The listing builds one solid part. Answer for the finished solid, in the listing's coordinates (mm). A direction names the side the tool comes from. Coordinates: 2 decimals unless noted, no trailing zeros. Order: outer loops, then holes, each group sorted by start corner. A loop starts at its lowest first (then second) coordinate and runs counter-clockwise, first axis right, second up. Notation, with made-up numbers: (51, 14.5) -> (60, 14.5) arc R17 ccw to (60, 42.5) -> close; hole circle Ø1 at (17.25, -37). An arc over 180 degrees is marked (long way). Put each result on its own line as item: value. Start each with the question number.
```python
from build123d import *

# Parameters (mm, degrees)
SALIENTE_EXTRUIR1_DEPTH                              = 100
CROQUIS3_W                                           = 20.92
CROQUIS3_H                                           = 92
CORTAR_EXTRUIR1_DEPTH                                = 798
CROQUIS4_W                                           = 19.08
CROQUIS4_H                                           = 92
CROQUIS4_W_2                                         = 20.25
CORTAR_EXTRUIR2_DEPTH                                = 798
CROQUIS5_W                                           = 465.67
CROQUIS5_H                                           = 136.54
CORTAR_EXTRUIR3_DEPTH                                = 69
REFRENTADO_PARA_PERNO_CON_CABEZA_HEXAGON_D           = 10.5
REFRENTADO_PARA_PERNO_CON_CABEZA_HEXAGON_DEPTH       = 90
REFRENTADO_PARA_PERNO_CON_CABEZA_HEXAGON_CBORE_D     = 13
REFRENTADO_PARA_PERNO_CON_CABEZA_HEXAGON_CBORE_DEPTH = 6.85
REFRENTADO_PARA_PERNO_CON_CABEZA_HEXAGON_TIP         = 3.15451825
CROQUIS8_R                                           = 8.5
CORTAR_EXTRUIR4_DEPTH                                = 69
CORTAR_EXTRUIR5_DEPTH                                = 607
CORTAR_EXTRUIR6_START                                = -138.5400001
CORTAR_EXTRUIR6_DEPTH                                = 138.5400001
REDONDEO1_R                                          = 10
REDONDEO2_R                                          = 10
REDONDEO3_R                                          = 10
REDONDEO4_R                                          = 10
REDONDEO5_R                                          = 10
CHAFL_N1_SIZE                                        = 1
REDONDEO6_R                                          = 10
SALIENTE_EXTRUIR2_DEPTH                              = 61
CROQUIS12_R                                          = 6.5
CORTAR_EXTRUIR7_DEPTH                                = 61
CORTAR_EXTRUIR8_DEPTH                                = 630
CORTAR_EXTRUIR9_START                                = -630
CROQUIS14_R                                          = 8.5
CORTAR_EXTRUIR9_DEPTH                                = 630


# Read off the part's stored shape, not the designer's step: Cortar-Extruir6
# Some blends are built 0.0001 mm under size
with BuildPart() as part:
    # Croquis2 → Saliente-Extruir1 (new body)
    with BuildSketch(Plane(origin=(0, 0, 0), x_dir=(1, 0, 0), z_dir=(0, 1, 0))):
        Polygon((-10, 20.92), (-10, 181.28), (497, 181.28), (497, 14.25), (482, 14.25), (482, 0), (0, 0), (0, 20.92), align=None)
    extrude(amount=SALIENTE_EXTRUIR1_DEPTH)

    # Croquis3 → Cortar-Extruir1 (cut)
    with BuildSketch(Plane.ZY.offset(10)):
        Polygon((-181.28, 100), (-181.28, 8), (-159.46, 8), (-159.46, 100), (-159.605192294, 100), align=None)
        with Locations((-10.46, 54)):
            Rectangle(CROQUIS3_W, CROQUIS3_H)
    extrude(amount=-CORTAR_EXTRUIR1_DEPTH, mode=Mode.SUBTRACT)

    # Croquis4 → Cortar-Extruir2 (cut)
    with BuildSketch(Plane(origin=(0, 0, -159.46), x_dir=(-1, 0, 0), z_dir=(0, 0, -1))):
        with Locations((0.46, 54)):
            Rectangle(CROQUIS4_W, CROQUIS4_H)
        with Locations((-486.875, 54)):
            Rectangle(CROQUIS4_W_2, CROQUIS4_H)
    extrude(amount=-CORTAR_EXTRUIR2_DEPTH, mode=Mode.SUBTRACT)

    # Croquis5 → Cortar-Extruir3 (cut)
    with BuildSketch(Plane.XZ):
        with Locations((242.915, -90.19)):
            Rectangle(CROQUIS5_W, CROQUIS5_H)
    extrude(amount=-CORTAR_EXTRUIR3_DEPTH, mode=Mode.SUBTRACT)

    # Refrentado para perno con cabeza hexagonal de M101
    with Locations(Plane(origin=(-0.5, 8, -131.28), x_dir=(0, 0, 1), z_dir=(0, 1, 0))):
        with Locations((0, 0), (75.36, 0), (121.325, 30.5), (121.325, 140.5), (121.325, 257.25), (121.325, 368.25), (121.325, 467.5), (-40.125, 467.5), (-40.125, 368.25), (-40.125, 257.25), (-40.125, 140.5), (-40.125, 30.5)):
            CounterBoreHole(REFRENTADO_PARA_PERNO_CON_CABEZA_HEXAGON_D / 2, REFRENTADO_PARA_PERNO_CON_CABEZA_HEXAGON_CBORE_D / 2, REFRENTADO_PARA_PERNO_CON_CABEZA_HEXAGON_CBORE_DEPTH, depth=REFRENTADO_PARA_PERNO_CON_CABEZA_HEXAGON_DEPTH)
            with Locations((0, 0, -(REFRENTADO_PARA_PERNO_CON_CABEZA_HEXAGON_DEPTH + REFRENTADO_PARA_PERNO_CON_CABEZA_HEXAGON_TIP / 2))):  # 118° drill point
                Cone(0, REFRENTADO_PARA_PERNO_CON_CABEZA_HEXAGON_D / 2, REFRENTADO_PARA_PERNO_CON_CABEZA_HEXAGON_TIP, mode=Mode.SUBTRACT)

    # Croquis8 → Cortar-Extruir4 (cut)
    with BuildSketch(Plane(origin=(476.75, 0, 0), x_dir=(0, 0, -1), z_dir=(1, 0, 0))):
        with Locations((50.94, 22)):
            Circle(CROQUIS8_R)
        with Locations((136.94, 22)):
            Circle(CROQUIS8_R)
    extrude(amount=-CORTAR_EXTRUIR4_DEPTH, mode=Mode.SUBTRACT)

    # Croquis9 → Cortar-Extruir5 (cut)
    with BuildSketch(Plane(origin=(476.75, 0, 0), x_dir=(0, 0, -1), z_dir=(1, 0, 0))):
        with BuildLine():
            Line((20.92, 69), (20.92, 100))
            Line((20.92, 100), (69.776934001, 100))
            ThreePointArc((69.776934001, 100), (40.845981718, 91.596052461), (20.92, 69))
        make_face()
        with BuildLine():
            Line((110.603065999, 100), (159.46, 100))
            Line((159.46, 100), (159.46, 69))
            ThreePointArc((159.46, 69), (139.534018282, 91.596052461), (110.603065999, 100))
        make_face()
    extrude(amount=-CORTAR_EXTRUIR5_DEPTH, mode=Mode.SUBTRACT)

    # Cortar-Extruir6 outline → Cortar-Extruir6 (cut)
    with BuildSketch(Plane.XY.offset(-20.92).offset(CORTAR_EXTRUIR6_START)):
        with BuildLine():
            Line((476.75, 100), (444.284633839, 100))
            ThreePointArc((444.284633839, 100), (466.729009526, 91.005318547), (476.75, 69))
            Line((476.75, 69), (476.75, 100))
        make_face()
        with BuildLine():
            ThreePointArc((9.08, 69), (19.100990474, 91.005318547), (41.545366161, 100))
            Line((41.545366161, 100), (9.08, 100))
            Line((9.08, 100), (9.08, 69))
        make_face()
    extrude(amount=CORTAR_EXTRUIR6_DEPTH, mode=Mode.SUBTRACT)

    # Redondeo1
    redondeo1_edges = [part.edges().sort_by_distance(p)[0] for p in [
        (475.75, 69, -90.19),
        (242.915, 69, -158.46),
        (10.08, 69, -90.19),
        (242.915, 69, -21.92),
    ]]
    fillet(redondeo1_edges, radius=REDONDEO1_R)

    # Redondeo2
    # the kernel refuses this fillet: 10 mm, written as the material it adds along each edge
    with BuildSketch(Plane(origin=(20.08, 59, -31.92), x_dir=(-1, 0, 0), z_dir=(0, 0, 1))) as redondeo2_piece_1_section:
        Polygon((0, 0), (REDONDEO2_R, 0), (REDONDEO2_R, -REDONDEO2_R), (0, -REDONDEO2_R), align=None)
    redondeo2_piece_1 = extrude(amount=REDONDEO2_R, mode=Mode.PRIVATE)
    redondeo2_piece_1 = redondeo2_piece_1 - Plane(origin=(20.08, 59, -31.92), x_dir=(0.7071067811865475, -0.7071067811865475, 0), z_dir=(0, 0, 1)) * Sphere(REDONDEO2_R, mode=Mode.PRIVATE)
    add(redondeo2_piece_1)
    with BuildSketch(Plane(origin=(10.08, 0, -21.92), x_dir=(1, 0, 0), z_dir=(0, 1, 0))) as redondeo2_piece_2:
        with BuildLine():
            CenterArc((REDONDEO2_R, REDONDEO2_R), REDONDEO2_R, 180, 90)
            Line((0, REDONDEO2_R), (0, 0))
            Line((0, 0), (REDONDEO2_R, 0))
        make_face()
    extrude(amount=59)

    # Redondeo3
    # the kernel refuses this fillet: 10 mm, written as the material it adds along each edge
    with BuildSketch(Plane(origin=(465.75, 59, -31.92), x_dir=(1, 0, 0), z_dir=(0, 0, 1))) as redondeo3_piece_1_section:
        Polygon((0, 0), (REDONDEO3_R, 0), (REDONDEO3_R, REDONDEO3_R), (0, REDONDEO3_R), align=None)
    redondeo3_piece_1 = extrude(amount=REDONDEO3_R, mode=Mode.PRIVATE)
    redondeo3_piece_1 = redondeo3_piece_1 - Plane(origin=(465.75, 59, -31.92), x_dir=(-0.7071067811865475, -0.7071067811865475, 0), z_dir=(0, 0, 1)) * Sphere(REDONDEO3_R, mode=Mode.PRIVATE)
    add(redondeo3_piece_1)
    with BuildSketch(Plane(origin=(475.75, 0, -21.92), x_dir=(-1, 0, 0), z_dir=(0, 1, 0))) as redondeo3_piece_2:
        with BuildLine():
            CenterArc((REDONDEO3_R, -REDONDEO3_R), REDONDEO3_R, 90, 90)
            Line((0, -REDONDEO3_R), (0, 0))
            Line((0, 0), (REDONDEO3_R, 0))
        make_face()
    extrude(amount=59)

    # Redondeo4
    # the kernel refuses this fillet: 10 mm, written as the material it adds along each edge
    with BuildSketch(Plane(origin=(465.75, 59, -148.46), x_dir=(0, 0, -1), z_dir=(1, 0, 0))) as redondeo4_piece_1_section:
        Polygon((0, 0), (REDONDEO4_R, 0), (REDONDEO4_R, REDONDEO4_R), (0, REDONDEO4_R), align=None)
    redondeo4_piece_1 = extrude(amount=REDONDEO4_R, mode=Mode.PRIVATE)
    redondeo4_piece_1 = redondeo4_piece_1 - Plane(origin=(465.75, 59, -148.46), x_dir=(0, -0.7071067811865475, 0.7071067811865475), z_dir=(1, 0, 0)) * Sphere(REDONDEO4_R, mode=Mode.PRIVATE)
    add(redondeo4_piece_1)
    with BuildSketch(Plane(origin=(475.75, 0, -158.46), x_dir=(0, 0, 1), z_dir=(0, 1, 0))) as redondeo4_piece_2:
        with BuildLine():
            CenterArc((REDONDEO4_R, -REDONDEO4_R), REDONDEO4_R, 90, 90)
            Line((0, -REDONDEO4_R), (0, 0))
            Line((0, 0), (REDONDEO4_R, 0))
        make_face()
    extrude(amount=59)

    # Redondeo5
    # the kernel refuses this fillet: 10 mm, written as the material it adds along each edge
    with BuildSketch(Plane(origin=(20.08, 59, -148.46), x_dir=(-1, 0, 0), z_dir=(0, 0, -1))) as redondeo5_piece_1_section:
        Polygon((0, 0), (REDONDEO5_R, 0), (REDONDEO5_R, REDONDEO5_R), (0, REDONDEO5_R), align=None)
    redondeo5_piece_1 = extrude(amount=REDONDEO5_R, mode=Mode.PRIVATE)
    redondeo5_piece_1 = redondeo5_piece_1 - Plane(origin=(20.08, 59, -148.46), x_dir=(0.7071067811865475, -0.7071067811865475, 0), z_dir=(0, 0, -1)) * Sphere(REDONDEO5_R, mode=Mode.PRIVATE)
    add(redondeo5_piece_1)
    with BuildSketch(Plane(origin=(10.08, 0, -158.46), x_dir=(1, 0, 0), z_dir=(0, 1, 0))) as redondeo5_piece_2:
        with BuildLine():
            CenterArc((REDONDEO5_R, -REDONDEO5_R), REDONDEO5_R, 90, 90)
            Line((0, -REDONDEO5_R), (0, 0))
            Line((0, 0), (REDONDEO5_R, 0))
        make_face()
    extrude(amount=59)

    # Chaflán1
    chafl_n1_edges = [part.edges().sort_by_distance(p)[0] for p in [
        (475.75, 22, -42.44),
        (475.75, 22, -128.44),
    ]]
    chamfer(chafl_n1_edges, length=CHAFL_N1_SIZE - 0.0001)  # a hair under: the kernel refuses the full size

    # Redondeo6
    redondeo6_edges = [part.edges().sort_by_distance(p)[0] for p in [
        (9.08, 38.5, -20.92),
        (9.08, 38.5, -159.46),
        (476.75, 38.5, -20.92),
        (476.75, 38.5, -159.46),
    ]]
    fillet(redondeo6_edges, radius=REDONDEO6_R)

    # Croquis11 → Saliente-Extruir2 (add)
    with BuildSketch(Plane(origin=(0, 8, 0), x_dir=(1, 0, 0), z_dir=(0, 1, 0))):
        Polygon((482, 0), (482, 14.25), (497, 14.25), (497, 181.28), (-10, 181.28), (-10, 20.92), (0, 20.92), (0, 0), align=None)
        with BuildLine():
            Line((466.75, 20.92), (19.08, 20.92))
            ThreePointArc((19.08, 20.92), (12.008932188, 23.848932188), (9.08, 30.92))
            Line((9.08, 30.92), (9.08, 149.46))
            ThreePointArc((9.08, 149.46), (12.008932188, 156.531067812), (19.08, 159.46))
            Line((19.08, 159.46), (466.75, 159.46))
            ThreePointArc((466.75, 159.46), (473.821067812, 156.531067812), (476.75, 149.46))
            Line((476.75, 149.46), (476.75, 30.92))
            ThreePointArc((476.75, 30.92), (473.821067812, 23.848932188), (466.75, 20.92))
        make_face(mode=Mode.SUBTRACT)
    extrude(amount=SALIENTE_EXTRUIR2_DEPTH)

    # Croquis12 → Cortar-Extruir7 (cut)
    with BuildSketch(Plane(origin=(0, 69, 0), x_dir=(1, 0, 0), z_dir=(0, 1, 0))):
        with Locations(Location((30, 171.405, 0), (0, 0, 270))):
            Circle(CROQUIS12_R)
        with Locations(Location((-0.5, 131.28, 0), (0, 0, 270))):
            Circle(CROQUIS12_R)
        with Locations(Location((256.75, 171.405, 0), (0, 0, 270))):
            Circle(CROQUIS12_R)
        with Locations(Location((367.75, 171.405, 0), (0, 0, 270))):
            Circle(CROQUIS12_R)
        with Locations(Location((467, 171.405, 0), (0, 0, 270))):
            Circle(CROQUIS12_R)
        with Locations(Location((467, 9.955, 0), (0, 0, 270))):
            Circle(CROQUIS12_R)
        with Locations(Location((367.75, 9.955, 0), (0, 0, 270))):
            Circle(CROQUIS12_R)
        with Locations(Location((256.75, 9.955, 0), (0, 0, 270))):
            Circle(CROQUIS12_R)
        with Locations(Location((140, 9.955, 0), (0, 0, 270))):
            Circle(CROQUIS12_R)
        with Locations(Location((30, 9.955, 0), (0, 0, 270))):
            Circle(CROQUIS12_R)
        with Locations(Location((140, 171.405, 0), (0, 0, 270))):
            Circle(CROQUIS12_R)
        with Locations(Location((-0.5, 55.92, 0), (0, 0, 270))):
            Circle(CROQUIS12_R)
    extrude(amount=-CORTAR_EXTRUIR7_DEPTH, mode=Mode.SUBTRACT)

    # Croquis13 → Cortar-Extruir8 (cut)
    with BuildSketch(Plane.ZY.offset(10)):
        Polygon((-181.28, 8), (-171.405, 69), (-181.28, 69), align=None)
        Polygon((0, 8), (-9.955, 69), (0, 69), align=None)
    extrude(amount=-CORTAR_EXTRUIR8_DEPTH, mode=Mode.SUBTRACT)

    # Croquis14 → Cortar-Extruir9 (cut)
    with BuildSketch(Plane.ZY.offset(-476.75).offset(CORTAR_EXTRUIR9_START)):
        with Locations((-136.94, 22)):
            Circle(CROQUIS14_R)
        with Locations((-50.94, 22)):
            Circle(CROQUIS14_R)
    extrude(amount=CORTAR_EXTRUIR9_DEPTH, mode=Mode.SUBTRACT)


solid = part.part
```
(1) A tool of negligible diameter and unlimited length cuts with its end or side. For faces 4 (the cylindrical face through (470.548, 0.567, -167.536)), 5 (the flat face through (10.08, 29, -91)), 6 (the cylindrical face through (369.702, 28.011, -165.205)), 7 (the cylindrical face through (475, 71.34, -155.11)), from which of +Z, -Z, +X, -X, +Y, -Y can it reach the whole face along a straight path? Write none if from no direction.
(2) For a pull along Y with two mould halves and no side action, classify faces 1 (the cylindrical face through (487.02, 30.48, -136.38)), 2 (the flat face through (240, 69, -89)), 3 (the flat face through (-10, 34, -102)) as released by +Y, released by -Y, zero draft, split by the parting line, or undercut.
(3) The part is cut by section B-B on x = 243. Determine the outline of the cut face in (y, z) (3 decimals), plus the area to 3 significant figures.
(4) Find the intervals of material crossed by L1, parallel to Z at x = 256.75, y = 0.5 (3 decimals); L2, parallel to Z at x = 467, y = 0.3 (3 decimals); L3, parallel to X at y = 21, z = -64, in increasing order.
(5) Each of these flat-tipped pins is pushed along its axis until it touches: P1, Ø1, axis at x = 212.5, z = -67, coming from the -Y side; P2, Ø6.5, axis at x = 465.5, z = -172, coming from the +Y side; P3, Ø16.5, axis at x = 489, y = 48, coming from the +Z side; P4, Ø14.5, axis at x = 469, z = -6.5, coming from the +Y side. Where does it stop, or does it pass through?
(6) The part is cut by section A-A on z = -97. Determine the outline of the cut face in (x, y), plus the area to 3 significant figures.
(7) The part is cut by section D-D on y = 94.5. Determine the outline of the cut face in (x, z), plus the area to 3 significant figures.
(8) The part is cut by section C-C on x = 367.75. Count the separate pieces of the cut face and the enclosed holes in it, plus the area to 3 significant figures.
Worked out:
1. face 4: +Y, -Y
1. face 5: -Y
1. face 6: +Y
1. face 7: -Z, +X, +Y
2. face 1: undercut
2. face 2: released by -Y
2. face 3: zero draft
3. outline: (0, -181.28) -> (8, -181.28) -> (69, -171.405) -> (69, -159.46) arc R54 ccw to (100, -110.603) -> (100, -69.777) arc R54 ccw to (69, -20.92) -> (69, -9.955) -> (8, 0) -> (0, 0) -> (0, -21.92) -> (59, -21.92) arc R10 cw to (69, -31.92) -> (69, -148.46) arc R10 cw to (59, -158.46) -> (0, -158.46) -> close
3. area: 5,960 mm2
4. L1: -181.28 to -176.655, -166.155 to -158.46, -21.92 to -15.205, -4.705 to 0
4. L2: -181.28 to -176.655, -166.155 to -158.382, -21.998 to -15.205, -4.705 to 0
4. L3: -10 to 10.08, 475.75 to 497
5. P1: y = 69
5. P2: through
5. P3: z = -5.82
5. P4: y = 69
6. outline: (-10, 0) -> (10.08, 0) -> (10.08, 59) arc R10 cw to (20.08, 69) -> (465.75, 69) arc R10 cw to (475.75, 59) -> (475.75, 0) -> (497, 0) -> (497, 69) -> (476.75, 69) arc R32.5 ccw to (444.28, 100) -> (41.55, 100) arc R32.5 ccw to (9.08, 69) -> (-10, 69) -> close
6. area: 16,900 mm2
7. outline: (23.46, -134.35) -> (462.37, -134.35) -> (462.37, -46.03) -> (23.46, -46.03) -> close
7. area: 38,800 mm2
8. separate pieces: 3
8. enclosed holes: 0
8. area: 4,440 mm2
